Solid Edge part; units mm, degrees
sketch "Sketch1" plane through (0, 0, 0) normal (0, 0, 1) x (1, 0, 0)
  circle A0 centre (0, 0) radius 3.5
extrude "Protrusion1" add sketch "Sketch1" along normal blind 4
sketch "Sketch2" plane through (0, 0, 0) normal (0, 0, -1) x (1, 0, 0)
  line L0 (0.85, 1.4722) -> (1.7, 0)
  line L1 (1.7, 0) -> (0.85, -1.4722)
  line L2 (0.85, -1.4722) -> (-0.85, -1.4722)
  line L3 (-0.85, -1.4722) -> (-1.7, 0)
  line L4 (-1.7, 0) -> (-0.85, 1.4722)
  line L5 (-0.85, 1.4722) -> (0.85, 1.4722)
extrude "ExtrudedCutout_1" cut sketch "Sketch2" against normal blind 2.4
sketch "Sketch3" plane through (0, 0, 4) normal (0, 0, 1) x (-1, 0, 0)
  circle A0 centre (0, 0) radius 2
extrude "ExtrudedProtrusion_2" add sketch "Sketch3" along normal blind 55
cosmetic_thread "Thread_2" thread depth 20
properties material "Stainless steel"
The listing builds one solid part. Answer for the finished solid, in the listing's coordinates (mm). A direction names the side the tool comes from. Give positions to 0.01 mm unless a question says otherwise; leave off trailing zeros. Loops run counter-clockwise (first coordinate to the right, second up) from the corner with the lowest first, then second, coordinate; pieces in that order, holes last.
Item 1: A cutting plane is placed at C-C (z = 45). Give the vertices of the cut face in (x, y).
Derived:
outline: circle Ø4 at (0, 0)
Item 2: A tool of negligible diameter and unlimited length cuts with its end or side. For faces 5 (the flat face through (0, -2, 0)), 6 (the cylindrical face through (0, -2, 31)), 7 (the flat face through (1.269, -0.746, 1.183)), from which of +Z, -Z, +X, -X, +Y, -Y can it reach the whole face along a straight path? Write none if from no direction.
Derived:
face 5: -Z, +X, -X, +Y, -Y
face 6: +Z
face 7: -Z
Item 3: A cutting plane is placed at D-D (y = -3). Give the vertices of the cut face in (x, z), then the cut area to 3 significant figures.
Derived:
outline: (-1.8, 0) - (1.8, 0) - (1.8, 4) - (-1.8, 4) - close
area: 14.4 mm2
Item 4: Determine the mould class of faces 1 (the flat face through (0, 0, 2.4)), 2 (the flat face through (0, 0, 59)), 3 (the cylindrical face through (3.233, 1.341, 1.972)), 4 (the flat face through (1.28, 0.73, 1.18)) for opening direction Y: +Y half, -Y half, draft (parallel to the pull), parting line (faces both ways), or undercut.
Derived:
face 1: undercut
face 2: draft
face 3: parting line
face 4: undercut
Item 5: Each of these flat-tipped pins is pushed along its axis until it touches: pin 1 Ø1 at (x, z) = (2, 47.5) entering from -Y; pin 2 Ø1.5 at (x, y) = (-2.5, -0.5) entering from +Z; pin 3 Ø3 at (x, z) = (0.5, 14.5) entering from -Y. Where does it stop, or does it pass through?
Derived:
pin 1: stops at y = -1.32
pin 2: stops at z = 59
pin 3: stops at y = -2
Item 6: A cutting plane is placed at B-B (y = -0.5). Give the vertices of the cut face in (x, z).
Derived:
outline: (-3.46, 0) - (-1.41, 0) - (-1.41, 2.4) - (1.41, 2.4) - (1.41, 0) - (3.46, 0) - (3.46, 4) - (1.94, 4) - (1.94, 59) - (-1.94, 59) - (-1.94, 4) - (-3.46, 4) - close
Item 7: A cutting plane is placed at A-A (x = 0). Give the vertices of the cut face in (y, z).
Derived:
outline: (-3.5, 0) - (-1.47, 0) - (-1.47, 2.4) - (1.47, 2.4) - (1.47, 0) - (3.5, 0) - (3.5, 4) - (2, 4) - (2, 59) - (-2, 59) - (-2, 4) - (-3.5, 4) - close
Item 8: Find the intervals of material crossed by line 1 along X through (y, z) = (0, 32.5); line 2 along Z through (x, y) = (-0.5, 2.75); line 3 along X through (y, z) = (0.25, 3), in increasing order.
Derived:
line 1: x = -2 to 2
line 2: z = 0 to 4
line 3: x = -3.49 to 3.49
